Model file for the job. Use its own axes, mm. A direction names the side the tool comes from. Round coordinates to 2 decimals unless told otherwise and drop trailing zeros. Loops run counter-clockwise (first coordinate to the right, second up) from the corner with the lowest first, then second, coordinate; pieces in that order, holes last. Notation, with made-up numbers: M 6.5,7.5 L 65.5,7.5 A33 ccw 65.5,44.5 Z; hole C 75,76.25 d8. An arc over 180 degrees is marked long. Answer in a Markdown table with one row per item.
from build123d import *

# Parameters (mm, degrees)
SKETCH1_W           = 50.2
SKETCH1_H           = 36.2
BOSS_EXTRUDE1_DEPTH = 1.5
SKETCH2_W           = 6.2
SKETCH2_H           = 1.5
BOSS_EXTRUDE2_DEPTH = 3
BOSS_EXTRUDE3_DEPTH = 1.5
SKETCH5_R           = 2.25
CUT_EXTRUDE1_DEPTH  = 1
SKETCH6_R           = 0.6
CUT_EXTRUDE2_DEPTH  = 1
SKETCH9_W           = 6.2
SKETCH9_H           = 4
BOSS_EXTRUDE4_DEPTH = 1.5


with BuildPart() as part:
    # Sketch1 → Boss-Extrude1 (new body)
    with BuildSketch(Plane(origin=(0, 0, 0), x_dir=(1, 0, 0), z_dir=(0, 1, 0))):
        with Locations((-25.1, -18.1)):
            Rectangle(SKETCH1_W, SKETCH1_H)
    extrude(amount=BOSS_EXTRUDE1_DEPTH)

    # Sketch2 → Boss-Extrude2 (add)
    with BuildSketch(Plane.XY.offset(36.2)):
        with Locations((-39.1, 0.75)):
            Rectangle(SKETCH2_W, SKETCH2_H)
        with Locations((-11.1, 0.75)):
            Rectangle(SKETCH2_W, SKETCH2_H)
    extrude(amount=BOSS_EXTRUDE2_DEPTH)

    # Sketch4 → Boss-Extrude3 (add)
    with BuildSketch(Plane(origin=(0, 1.5, 0), x_dir=(1, 0, 0), z_dir=(0, 1, 0))):
        with BuildLine():
            Line((-32.69, 0), (-17.51, 0))
            ThreePointArc((-17.51, 0), (-25.1, 7.59), (-32.69, 0))
        make_face()
    extrude(amount=-BOSS_EXTRUDE3_DEPTH)

    # Sketch5 → Cut-Extrude1 (cut)
    with BuildSketch(Plane(origin=(0, 1.5, 0), x_dir=(1, 0, 0), z_dir=(0, 1, 0))):
        with Locations((-25.1, 3.4)):
            Circle(SKETCH5_R)
    extrude(amount=-CUT_EXTRUDE1_DEPTH, mode=Mode.SUBTRACT)

    # Sketch6 → Cut-Extrude2 (cut)
    with BuildSketch(Plane(origin=(0, 0.5, 0), x_dir=(1, 0, 0), z_dir=(0, 1, 0))):
        with Locations((-25.1, 3.4)):
            Circle(SKETCH6_R)
    extrude(amount=-CUT_EXTRUDE2_DEPTH, mode=Mode.SUBTRACT)

    # Sketch9 → Boss-Extrude4 (add)
    with BuildSketch(Plane.XZ):
        with Locations((-39.1, 39.1)):
            Rectangle(SKETCH9_W, SKETCH9_H)
        with Locations((-11.1, 39.1)):
            Rectangle(SKETCH9_W, SKETCH9_H)
    extrude(amount=BOSS_EXTRUDE4_DEPTH)


solid = part.part
1. Saw through at A-A (x = -25.1). Write the cut outline in (y, z), and give its area (3 significant figures).
Verdict:
| item | result |
|---|---|
| outline | M 0,-7.59 L 1.5,-7.59 L 1.5,-5.65 L 0.5,-5.65 L 0.5,-4 L 0,-4 Z; M 0,-2.8 L 0.5,-2.8 L 0.5,-1.15 L 1.5,-1.15 L 1.5,36.2 L 0,36.2 Z |
| area | 60.6 mm² |
2. Pin check, flat tips, straight feed: pin 1 (1.6 mm diameter, centred on x = -11.5, y = -1, fed in from -Z); pin 2 (7 mm diameter, centred on x = -25.1, z = -3.4, fed in from -Y); pin 3 (1.2 mm diameter, centred on x = -12.5, y = 1, fed in from -Z); pin 4 (1.1 mm diameter, centred on x = -25.1, z = -3.4, fed in from +Y). Stop position of each tip, or through.
Verdict:
| item | result |
|---|---|
| pin 1 | stops at z = 37.1 |
| pin 2 | stops at y = 0 |
| pin 3 | stops at z = 0 |
| pin 4 | passes through |
3. Tool access for faces 1 (the flat face through (-42.2, 0, 39)), 2 (the flat face through (-25, 0, 19)), 3 (the flat face through (-26, 0.5, -3)), 4 (the flat face through (-39, 0, 40)), 5 (the flat face through (-42, 1, 0)): list every direction of +Z, -Z, +X, -X, +Y, -Y with a clear straight run to the whole face (end or side of a thin tool).
Verdict:
| item | result |
|---|---|
| face 1 | +Z, -X, +Y, -Y |
| face 2 | -Z, +X, -X, -Y |
| face 3 | +Y |
| face 4 | +Z, +X, -X, +Y |
| face 5 | -Z, -X, +Y, -Y |
4. Saw through at B-B (y = -0.65). Write the cut outline in (x, z).
Verdict:
| item | result |
|---|---|
| outline | M -42.2,37.1 L -36,37.1 L -36,41.1 L -42.2,41.1 Z; M -14.2,37.1 L -8,37.1 L -8,41.1 L -14.2,41.1 Z |
5. Wall check: probe 1 along Z at (x, y) = (-25.1, 0.15); probe 2 along Z at (x, y) = (-25.1, 0.9); probe 3 along Y at (x, z) = (-39, 17.5). Give the ranges that are in metal, low to high.
Verdict:
| item | result |
|---|---|
| probe 1 | z = -7.59 to -4, -2.8 to 36.2 |
| probe 2 | z = -7.59 to -5.65, -1.15 to 36.2 |
| probe 3 | y = 0 to 1.5 |
6. Saw through at D-D (x = -38). Write the cut outline in (y, z).
Verdict:
| item | result |
|---|---|
| outline | M -1.5,37.1 L 0,37.1 L 0,0 L 1.5,0 L 1.5,39.2 L 0,39.2 L 0,41.1 L -1.5,41.1 Z |
7. Saw through at C-C (z = -3.4). Write the cut outline in (x, y), and give its area (3 significant figures).
Verdict:
| item | result |
|---|---|
| outline | M -31.89,0 L -25.7,0 L -25.7,0.5 L -27.35,0.5 L -27.35,1.5 L -31.89,1.5 Z; M -24.5,0 L -18.31,0 L -18.31,1.5 L -22.85,1.5 L -22.85,0.5 L -24.5,0.5 Z |
| area | 15.3 mm² |
8. Mould opens along X. For faces 6 (the flat face through (-25, 1, 36.2)), 7 (the flat face through (0, 1, 18)), 8 (the flat face through (-50.2, 1, 18)) say: +X half, -X half, draft (parallel to the pull), parting line (faces both ways), or undercut.
Verdict:
| item | result |
|---|---|
| face 6 | undercut |
| face 7 | +X half |
| face 8 | -X half |
